Can you work these out from the drawing? Everything is in mm from the part's minimum corner. A direction names the side the tool comes from. Coordinates: 2 decimals unless noted, no trailing zeros. Order: outer loops, then holes, each group sorted by start corner. A loop starts at its lowest first (then second) coordinate and runs counter-clockwise, first axis right, second up. Notation, with made-up numbers: (47, -14.5) - (69, -14.5) arc R15 cw to (69, 4.5) - close; hole circle Ø8 at (67, 16.5). An arc over 180 degrees is marked (long way). Use a Markdown table: item, result. Add a question column.
(1) I want a section at B-B (y = 11). List the corners of the cut face in (x, z) for me, and give its area (3 significant figures).
(2) I want a section at D-D (x = 21). List the corners of the cut face in (y, z) for me, and give its area (3 significant figures).
(3) I want a section at C-C (z = 8). List the corners of the cut face in (x, y) for me, and give its area (3 significant figures).
(4) I want a section at A-A (x = 93). List the corners of the cut face in (y, z) for me.
(5) On a 3-axis mill with a long thin cutter (end or side, diameter ignored), from which of +Z, -Z, +X, -X, +Y, -Y can I reach the whole of each face in a straight line? I mean the marked faces 1 and 2. Say none if no direction works.
(6) If I drill on L1, parallel to Y at x = 49, z = 19.1; L2, parallel to Y at x = 104.8, z = 8; L3, parallel to Y at x = 93, z = 18, over which ranges is the centre line in solid material (lowest first)? Write a range as [from, to].
(7) For pin 1 Ø1.5 at (y, z) = (45, 9) entering from +X; pin 2 Ø4 at (y, z) = (28.5, 12.5) entering from -X; pin 3 Ø4.5 at (x, z) = (12.5, 18) entering from +Y; pin 4 Ø6 at (x, y) = (93, 25) entering from -Z, each with a flat end and sliding along its axis, tell me the tip position at first contact or that it passes through.
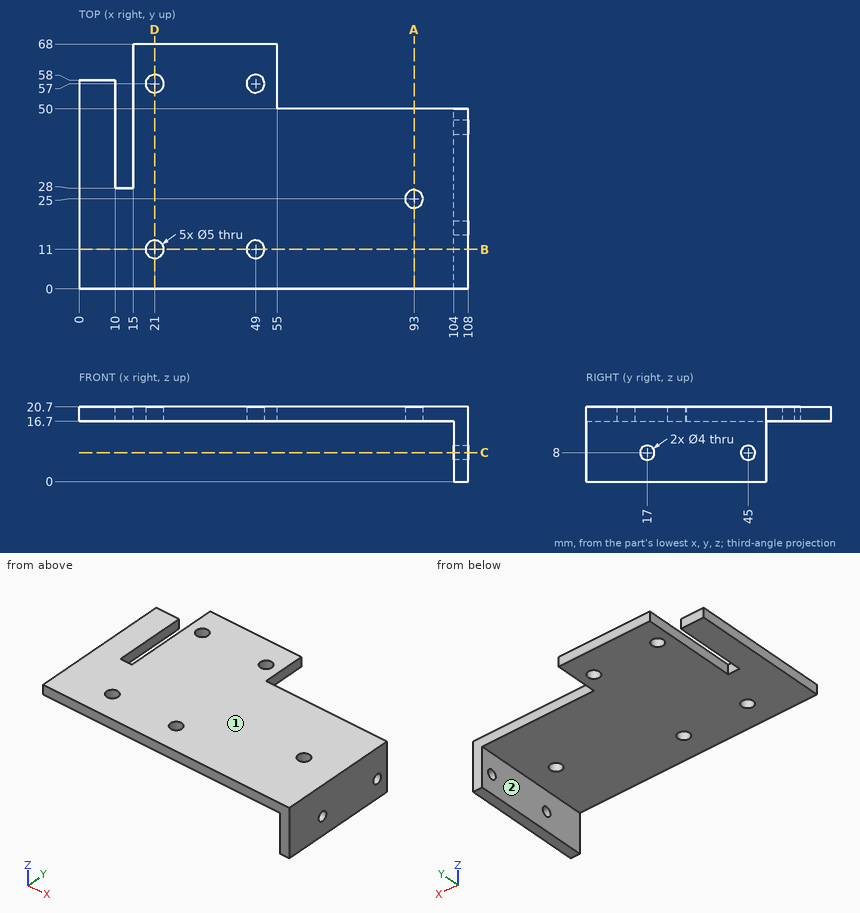
Answers follow:
| question | item | result |
|---|---|---|
| 1 | outline | (0, 16.7) - (18.5, 16.7) - (18.5, 20.7) - (0, 20.7) - close; (23.5, 16.7) - (46.5, 16.7) - (46.5, 20.7) - (23.5, 20.7) - close; (51.5, 16.7) - (104, 16.7) - (104, 0) - (108, 0) - (108, 20.7) - (51.5, 20.7) - close |
| 1 | area | 459 mm² |
| 2 | outline | (0, 16.7) - (8.5, 16.7) - (8.5, 20.7) - (0, 20.7) - close; (13.5, 16.7) - (54.5, 16.7) - (54.5, 20.7) - (13.5, 20.7) - close; (59.5, 16.7) - (68, 16.7) - (68, 20.7) - (59.5, 20.7) - close |
| 2 | area | 232 mm² |
| 3 | outline | (104, 0) - (108, 0) - (108, 15) - (104, 15) - close; (104, 19) - (108, 19) - (108, 43) - (104, 43) - close; (104, 47) - (108, 47) - (108, 50) - (104, 50) - close |
| 3 | area | 168 mm² |
| 4 | outline | (0, 16.7) - (22.5, 16.7) - (22.5, 20.7) - (0, 20.7) - close; (27.5, 16.7) - (50, 16.7) - (50, 20.7) - (27.5, 20.7) - close |
| 5 | face 1 | +Z, +X, -X, +Y, -Y |
| 5 | face 2 | -Z, -X, +Y, -Y |
| 6 | L1 | y = [0, 8.5], [13.5, 54.5], [59.5, 68] |
| 6 | L2 | y = [0, 15], [19, 43], [47, 50] |
| 6 | L3 | y = [0, 22.5], [27.5, 50] |
| 7 | pin 1 | passes through |
| 7 | pin 2 | stops at x = 104 |
| 7 | pin 3 | stops at y = 28 |
| 7 | pin 4 | stops at z = 16.7 |
